Can you work these out from the model? Positions are in its coordinate system, mm. A direction names the side the tool comes from. Give positions to 0.01 mm unless a question says otherwise; leave off trailing zeros. Order: outer loops, then holes, each group sorted by start corner. A loop starts at its lowest first (then second) coordinate and runs counter-clockwise, first axis right, second up.
Item 1: I want a section at C-C, the plane y = 3.5. Write out the boundary of the cut face in (x, z).
Item 2: If I drill on line 1 along Z through (x, y) = (-6.25, 11.25); line 2 along Z through (x, y) = (-2.25, 10.25); line 3 along Y through (x, z) = (-0.25, 18), over which ranges is the centre line in solid material (lowest first)?
Item 3: I want a section at B-B, the plane y = 1.25. Write out the boundary of the cut face in (x, z).
Item 4: Which directions (+Z, -Z, +X, -X, +Y, -Y) give clear straight access to the entire face, cutting with the end or side of a thin tool? Please do faces 1 (the flat face through (1.4, 12.4, 15.05)), 2 (the flat face through (0, 17.4, 0)).
Item 5: I want a section at A-A, the plane x = 0. Write out the boundary of the cut face in (y, z).
Item 6: I want a section at D-D, the plane x = 6. Write out the boundary of the cut face in (y, z).
```python
from build123d import *

# Parameters (mm, degrees)
SKETCH1_W           = 15.2
SKETCH1_H           = 30.1
BOSS_EXTRUDE1_DEPTH = 17.4
FILLET1_R           = 1
SKETCH3_R           = 5.35
BOSS_EXTRUDE2_DEPTH = 3.8
SKETCH4_R           = 5.25
BOSS_EXTRUDE3_DEPTH = 1.5
BOSS_EXTRUDE4_DEPTH = 3.8
BOSS_EXTRUDE4_TAPER = 4


with BuildPart() as part:
    # Sketch1 → Boss-Extrude1 (new body)
    with BuildSketch(Plane(origin=(0, 0, 0), x_dir=(1, 0, 0), z_dir=(0, 1, 0))):
        Rectangle(SKETCH1_W, SKETCH1_H)
    extrude(amount=BOSS_EXTRUDE1_DEPTH)

    # Fillet1
    fillet1_edges = [part.edges().sort_by_distance(p)[0] for p in [
        (-7.6, 8.7, -15.05),
        (7.6, 8.7, -15.05),
        (7.6, 8.7, 15.05),
        (-7.6, 8.7, 15.05),
    ]]
    fillet(fillet1_edges, radius=FILLET1_R)

    # Sketch3 → Boss-Extrude2 (add)
    with BuildSketch(Plane.XY.offset(15.05)):
        with Locations((0, 7.030745518)):
            Circle(SKETCH3_R)
    extrude(amount=BOSS_EXTRUDE2_DEPTH)

    # Sketch4 → Boss-Extrude3 (add)
    with BuildSketch(Plane.XY.offset(18.85)):
        with Locations((0, 7.030745518)):
            Circle(SKETCH4_R)
    extrude(amount=BOSS_EXTRUDE3_DEPTH)

    # Sketch5 → Boss-Extrude4 (add)
    with BuildSketch(Plane.XY.offset(20.35)):
        with BuildLine():
            ThreePointArc((-1.25, 9.380745518), (-3.6, 7.030745518), (-1.25, 4.680745518))
            Line((-1.25, 4.680745518), (1.25, 4.680745518))
            ThreePointArc((1.25, 4.680745518), (3.6, 7.030745518), (1.25, 9.380745518))
            Line((1.25, 9.380745518), (-1.25, 9.380745518))
        make_face()
    extrude(amount=BOSS_EXTRUDE4_DEPTH, taper=BOSS_EXTRUDE4_TAPER)


solid = part.part
```
Results list:
1. outline: (-7.6, -14.05) arc R1 ccw to (-6.6, -15.05) - (6.6, -15.05) arc R1 ccw to (7.6, -14.05) - (7.6, 14.05) arc R1 ccw to (6.6, 15.05) - (4.02, 15.05) - (4.02, 18.85) - (3.89, 18.85) - (3.89, 20.35) - (-3.89, 20.35) - (-3.89, 18.85) - (-4.02, 18.85) - (-4.02, 15.05) - (-6.6, 15.05) arc R1 ccw to (-7.6, 14.05) - close
2. line 1: z = -15.05 to 15.05
2. line 2: z = -15.05 to 20.35
2. line 3: y = 1.69 to 12.37
3. outline: (-7.6, -14.05) arc R1 ccw to (-6.6, -15.05) - (6.6, -15.05) arc R1 ccw to (7.6, -14.05) - (7.6, 14.05) arc R1 ccw to (6.6, 15.05) - (-6.6, 15.05) arc R1 ccw to (-7.6, 14.05) - close
4. face 1: +Z
4. face 2: +Z, -Z, +X, -X, +Y
5. outline: (0, -15.05) - (17.4, -15.05) - (17.4, 15.05) - (12.38, 15.05) - (12.38, 18.85) - (12.28, 18.85) - (12.28, 20.35) - (9.38, 20.35) - (9.12, 24.15) - (4.95, 24.15) - (4.68, 20.35) - (1.78, 20.35) - (1.78, 18.85) - (1.68, 18.85) - (1.68, 15.05) - (0, 15.05) - close
6. outline: (0, -15.05) - (17.4, -15.05) - (17.4, 15.05) - (0, 15.05) - close
